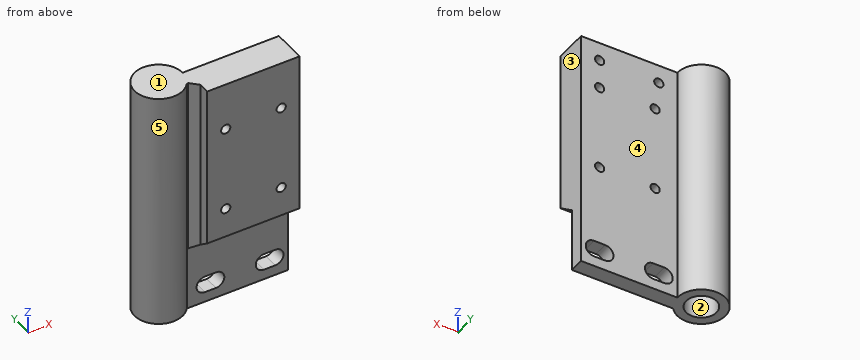
from build123d import *

# Parameters (mm, degrees)
SKETCH_1_R           = 4.1
EXTRUDE_1_DEPTH      = 65
SKETCH_2_R           = 4.923200542
EXTRUDE_2_DEPTH      = 3
SKETCH_3_R           = 1.25
CUT_EXTRUDE_1_DEPTH  = 13
EXTRUDE_3_DEPTH      = 12.5
EXTRUDE_3_DEPTH_BACK = 12.5
CHAMFER_4_SIZE       = 2
SKETCH_5_R           = 1.25
CUT_EXTRUDE_2_DEPTH  = 10


with BuildPart() as part:
    # Sketch 1 → Extrude 1 (new body)
    with BuildSketch(Plane.XY):
        with BuildLine():
            Line((5.123475383, -4), (32.5, -4))
            Line((32.5, -4), (32.5, 0))
            Line((32.5, 0), (6.5, 0))
            ThreePointArc((6.5, 0), (-6.146242348, 2.115113473), (5.123475383, -4))
        make_face()
        Circle(SKETCH_1_R, mode=Mode.SUBTRACT)
    extrude(amount=EXTRUDE_1_DEPTH)

    # Sketch 2 → Extrude 2 (add)
    with BuildSketch(Plane.XY.offset(65)):
        Circle(SKETCH_2_R)
    extrude(amount=-EXTRUDE_2_DEPTH)

    # Sketch 3 → Cut-Extrude 1 (cut)
    with BuildSketch(Plane(origin=(0, 0, 0), x_dir=(1, 0, 0), z_dir=(0, 1, 0))):
        with Locations((11.5, -60)):
            Circle(SKETCH_3_R)
        with Locations((27.5, -60)):
            Circle(SKETCH_3_R)
        with BuildLine():
            Line((10, -7.25), (13, -7.25))
            ThreePointArc((13, -7.25), (15.25, -5), (13, -2.75))
            Line((13, -2.75), (10, -2.75))
            ThreePointArc((10, -2.75), (7.75, -5), (10, -7.25))
        make_face()
        with BuildLine():
            Line((26, -2.75), (29, -2.75))
            ThreePointArc((29, -2.75), (31.25, -5), (29, -7.25))
            Line((29, -7.25), (26, -7.25))
            ThreePointArc((26, -7.25), (23.75, -5), (26, -2.75))
        make_face()
    extrude(amount=-CUT_EXTRUDE_1_DEPTH, mode=Mode.SUBTRACT)

    # Sketch 4 → Extrude 3 (add, two sides)
    with BuildSketch(Plane(origin=(20, 0, 0), x_dir=(0, 0, -1), z_dir=(1, 0, 0))) as extrude_3_sk:
        Polygon((-17.25, -4), (-21.094184264, -9), (-65, -9), (-65, -4), align=None)
    extrude(amount=EXTRUDE_3_DEPTH)
    extrude(extrude_3_sk.sketch, amount=-EXTRUDE_3_DEPTH_BACK)

    # Chamfer 4
    chamfer_4_edges = [part.edges().sort_by_distance(p)[0] for p in [
        (7.5, -4, 41.125),
    ]]
    chamfer(chamfer_4_edges, length=CHAMFER_4_SIZE)

    # Sketch 5 → Cut-Extrude 2 (cut)
    with BuildSketch(Plane.XZ.offset(9)):
        with Locations((27.5, 29.094184264)):
            Circle(SKETCH_5_R)
        with Locations((12.5, 29.094184264)):
            Circle(SKETCH_5_R)
        with Locations((27.5, 52.094184264)):
            Circle(SKETCH_5_R)
        with Locations((12.5, 52.094184264)):
            Circle(SKETCH_5_R)
    extrude(amount=-CUT_EXTRUDE_2_DEPTH, mode=Mode.SUBTRACT)


solid = part.part
Read the model definition and answer for the solid it produces. Units are mm, in the model's axes. Face numbers are marked on the shaded views. A direction names the side the tool comes from. Coordinates: 2 decimals unless noted, no trailing zeros. Loops run counter-clockwise (first coordinate to the right, second up) from the corner with the lowest first, then second, coordinate; pieces in that order, holes last. Notation, with made-up numbers: (-12, 6.25) - (23, 6.25) arc R30 cw to (23, 43.25) - close; hole circle Ø6 at (88.25, 88.5). An arc over 180 degrees is marked (long way). Answer in a Markdown table with one row per item.
Q1. Straight lines are drawn through the part: line 1 along Y through (x, z) = (0, 33); line 2 along Z through (x, y) = (11.5, -3.05); line 3 along Z through (x, y) = (27.5, -7). For each, find the intervals that lie inside material, in ascending order. Write a range as [from, to].
Here are the results:
| item | result |
|---|---|
| line 1 | y = [-6.5, -4.1], [4.1, 6.5] |
| line 2 | z = [0, 2.75], [7.25, 28.34], [29.84, 51.34], [52.84, 58.75], [61.25, 65] |
| line 3 | z = [19.56, 27.84], [30.34, 50.84], [53.34, 65] |
Q2. Find section A-A on x = 27.5. Write down the section's boundary in (y, z), plus the area to 3 significant figures.
Here are the results:
| item | result |
|---|---|
| outline | (-9, 21.09) - (-4, 17.25) - (-4, 7.25) - (0, 7.25) - (0, 27.84) - (-9, 27.84) - close; (-9, 30.34) - (0, 30.34) - (0, 50.84) - (-9, 50.84) - close; (-9, 53.34) - (0, 53.34) - (0, 58.75) - (-4, 58.75) - (-4, 61.25) - (0, 61.25) - (0, 65) - (-9, 65) - close; (-4, 0) - (0, 0) - (0, 2.75) - (-4, 2.75) - close |
| area | 416 mm^2 |
Q3. For the marked faces 4 and 5, determine the directions among +Z, -Z, +X, -X, +Y, -Y from which every point of the face is accessible in a straight line to the end or side of a thin tool.
Here are the results:
| item | result |
|---|---|
| face 4 | +Z, -Z, +X, +Y |
| face 5 | +Z, -Z |
Q4. Find section B-B on y = -5.25. Write down the section's boundary in (x, z), plus the area to 3 significant figures.
Here are the results:
| item | result |
|---|---|
| outline | (-3.83, 0) - (3.83, 0) - (3.83, 65) - (-3.83, 65) - close; (6.75, 18.21) - (32.5, 18.21) - (32.5, 65) - (6.75, 65) - close; hole circle Ø2.5 at (12.5, 29.09); hole circle Ø2.5 at (12.5, 52.09); hole circle Ø2.5 at (27.5, 29.09); hole circle Ø2.5 at (27.5, 52.09) |
| area | 1,680 mm^2 |
Q5. The mould has two halves that part along X. Classify the marked faces 1, 2 and 3: pulls with the +X half, pulls with the -X half, needs draft (parallel to the pull), parting line crosses it, or undercut.
Here are the results:
| item | result |
|---|---|
| face 1 | needs draft |
| face 2 | undercut |
| face 3 | pulls with the +X half |
Q6. Find section C-C on z = 60. Write down the section's boundary in (x, y).
Here are the results:
| item | result |
|---|---|
| outline | (5.12, -4) - (5.5, -4) - (7.5, -6) - (7.5, -9) - (32.5, -9) - (32.5, 0) - (28.75, 0) - (28.75, -4) - (26.25, -4) - (26.25, 0) - (12.75, 0) - (12.75, -4) - (10.25, -4) - (10.25, 0) - (6.5, 0) arc R6.5 ccw (long way) to start; hole circle Ø8.2 at (0, 0) |
Q7. Given P1, Ø4, axis at x = 11.5, z = 60, coming from the +Y side; P2, Ø2, axis at x = 27.5, z = 60, coming from the +Y side; P3, Ø3, axis at x = 3, z = 12.5, coming from the +Y side, each flat-ended and moving along its own axis, determine where each tip first touches the part or whether it passes through.
Here are the results:
| item | result |
|---|---|
| P1 | stops at y = 0 |
| P2 | stops at y = -4 |
| P3 | stops at y = 6.32 |
Q8. Find section D-D on x = 16. Write down the section's boundary in (y, z), plus the area to 3 significant figures.
Here are the results:
| item | result |
|---|---|
| outline | (-9, 21.09) - (-4, 17.25) - (-4, 0) - (0, 0) - (0, 65) - (-9, 65) - close |
| area | 489 mm^2 |
